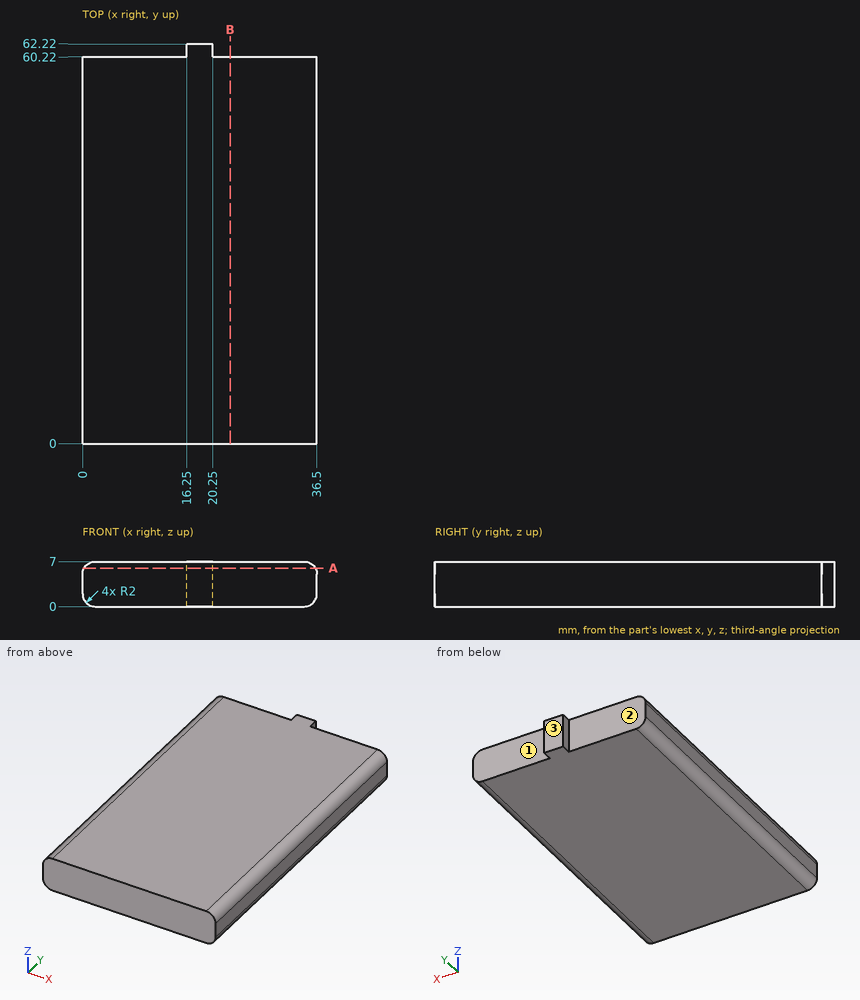
Check sheet for the drawn part. Datum: minimum x, y, z corner. Units: mm. A direction names the side the tool comes from. Give positions to 0.01 mm unless a question says otherwise; leave off trailing zeros. Write each loop counter-clockwise with the first axis right and the second up, starting at its lowest first coordinate (ties: lowest second). Pieces come first, ordered by that corner, then holes. Notation, with made-up numbers: M 72.25,7 L 85.25,7 A29 cw 85.25,46 Z; hole C -1.75,1.25 d7. An arc over 180 degrees is marked long. One line per question, with ' | ' between items.
1) Gauge pin test, flat ends, axial feed: pin 1 Ø1.5 at (x, z) = (14, 6) entering from +Y; pin 2 Ø1 at (y, z) = (26.5, 1) entering from -X; pin 3 Ø0.6 at (y, z) = (61.5, 3.5) entering from -X. Record the tip position at first contact, or that the pin passes through.
Result:
pin 1: stops at y = 60.22 | pin 2: stops at x = 0.06 | pin 3: stops at x = 16.25
2) Set-up check for the marked faces 1, 2 and 3: record each of +Z, -Z, +X, -X, +Y, -Y from which the full face is reachable in a straight line by a thin tool's end or side.
Result:
face 1: +Z, -Z, +X, +Y | face 2: +Z, -Z, -X, +Y | face 3: +Z, -Z, +X, -X, +Y
3) Section check B-B on x = 23. Enter the section's corners in (y, z).
Result:
outline: M 0,0 L 60.22,0 L 60.22,7 L 0,7 Z
4) Thickness scan on line 1 along Y through (x, z) = (13, 3.5); line 2 along Z through (x, y) = (35, 26.5); line 3 along X through (y, z) = (9.5, 1.5). Record the ranges inside material, lowest first. Write a range as [from, to].
Result:
line 1: y = [0, 60.22] | line 2: z = [0.06, 6.94] | line 3: x = [0.06, 36.44]
5) Section check A-A on z = 6. Enter the section's corners in (x, y), plus the area to 3 significant figures.
Result:
outline: M 0.27,0 L 36.23,0 L 36.23,60.22 L 20.25,60.22 L 20.25,62.22 L 16.25,62.22 L 16.25,60.22 L 0.27,60.22 Z | area: 2,170 mm2
